Geometry: final body of the model. Coordinates: model frame, mm. Coordinates: 2 decimals unless noted, no trailing zeros. Write each loop counter-clockwise with the first axis right and the second up, starting at its lowest first coordinate (ties: lowest second). Pieces come first, ordered by that corner, then holes. Notation, with made-up numbers: (41, 23) - (51, 23) arc R30 ccw to (51, 61) - close; hole circle Ø10 at (-32, 52.5). An arc over 180 degrees is marked (long way). Put each result on its own line as item: value.
```python
from build123d import *

# Parameters (mm, degrees)
RESSALTO_EXTRUS_O1_DEPTH = 5
ESBO_O2_R                = 1.5
CORTE_EXTRUS_O1_DEPTH    = 10


with BuildPart() as part:
    # Esboço1 → Ressalto-extrusão1 (new body)
    with BuildSketch(Plane.XY):
        with BuildLine():
            Line((-16.520541228, -40.769230769), (3.479458772, -40.769230769))
            ThreePointArc((3.479458772, -40.769230769), (83.479458772, -120.769230769), (163.479458772, -40.769230769))
            Line((163.479458772, -40.769230769), (183.479458772, -40.769230769))
            ThreePointArc((183.479458772, -40.769230769), (157.119069078, -104.408841076), (93.479458772, -130.769230769))
            Line((93.479458772, -130.769230769), (73.479458772, -130.769230769))
            ThreePointArc((73.479458772, -130.769230769), (9.839848465, -104.408841076), (-16.520541228, -40.769230769))
        make_face()
    extrude(amount=RESSALTO_EXTRUS_O1_DEPTH)

    # Esboço2 → Corte-extrusão1 (cut)
    with BuildSketch(Plane.XY.offset(5)):
        with Locations((83.479458772, -125.769230769)):
            Circle(ESBO_O2_R)
        with Locations((148.479458772, -100.769230769)):
            Circle(ESBO_O2_R)
        with Locations((173.479458772, -60.769230769)):
            Circle(ESBO_O2_R)
        with Locations((-6.520541228, -60.769230769)):
            Circle(ESBO_O2_R)
        with Locations((18.479458772, -100.769230769)):
            Circle(ESBO_O2_R)
    extrude(amount=-CORTE_EXTRUS_O1_DEPTH, mode=Mode.SUBTRACT)


solid = part.part
```
1. Section query D-D (x = 53). Return loops of the section in (y, z).
Answer below:
outline: (-128.41, 0) - (-114.74, 0) - (-114.74, 5) - (-128.41, 5) - close
2. Section query A-A (y = -94.5). Return loops of the section in (x, z), then the cut area to 3 significant figures.
Answer below:
outline: (1.28, 0) - (24.21, 0) - (24.21, 5) - (1.28, 5) - close; (142.75, 0) - (165.68, 0) - (165.68, 5) - (142.75, 5) - close
area: 229 mm²
3. Ray query, probe 1 along X at (y, z) = (-102, 1.9); probe 2 along X at (y, z) = (-83.5, 1.8); probe 3 along X at (y, z) = (-58, 3.5). Return the intervals inside material, ascending. Write a range as from..to.
Answer below:
probe 1: x = 7.52..17.62, 19.34..31.99, 134.97..147.62, 149.34..159.44
probe 2: x = -5.73..15.85, 151.11..172.69
probe 3: x = -14.86..5.36, 161.6..181.81
4. Mould query, pull axis X, two halves, no side actions, for faces 1 (the flat face through (77, -122, 5)), 2 (the cylindrical face through (157.81, -103.71, 2.46)), 3 (the cylindrical face through (81.72, -120.75, 2.46)). Classes: +X half, -X half, draft (parallel to the pull), parting line (faces both ways), or undercut.
Answer below:
face 1: draft
face 2: +X half
face 3: undercut
5. Section query B-B (z = 3.75). Return loops of the section in (x, y), then the cut area to 4 significant figures.
Answer below:
outline: (-16.52, -40.77) arc R90 ccw to (73.48, -130.77) - (93.48, -130.77) arc R90 ccw to (183.48, -40.77) - (163.48, -40.77) arc R80 cw to (3.48, -40.77) - close; hole circle Ø3 at (-6.52, -60.77); hole circle Ø3 at (18.48, -100.77); hole circle Ø3 at (83.48, -125.77); hole circle Ø3 at (148.48, -100.77); hole circle Ø3 at (173.48, -60.77)
area: 4,435 mm²
6. Pin query (flat end, axial travel): pin 1 Ø1.8 at (x, y) = (-6.52, -60.77) entering from -Z; pin 2 Ø3 at (y, z) = (-115.5, 4) entering from +X; pin 3 Ø3 at (y, z) = (-88, 2) entering from -X; pin 4 Ø1 at (y, z) = (-109.5, 2.5) entering from +X. Return the tip coordinate at first contact, or that it passes through.
Answer below:
pin 1: passes through
pin 2: stops at x = 145.8
pin 3: stops at x = -4.04
pin 4: stops at x = 152.17
7. Section query C-C (y = -115.5). Return loops of the section in (x, z), then the cut area to 3 significant figures.
Answer below:
outline: (23.33, 0) - (54.93, 0) - (54.93, 5) - (23.33, 5) - close; (112.03, 0) - (143.63, 0) - (143.63, 5) - (112.03, 5) - close
area: 316 mm²
